```python
from build123d import *

# Parameters (mm, degrees)
SKETCH2_W           = 7.05
SKETCH2_H           = 26.75
BOSS_EXTRUDE1_DEPTH = 3.175
SKETCH3_W           = 7.05
SKETCH3_H           = 3.175
BOSS_EXTRUDE2_DEPTH = 20
SKETCH4_R           = 2.25
CUT_EXTRUDE1_DEPTH  = 3.175
SKETCH5_R           = 2.15
CUT_EXTRUDE2_DEPTH  = 34.585534461


with BuildPart() as part:
    # Sketch2 → Boss-Extrude1 (new body)
    with BuildSketch(Plane(origin=(0, 0, 0), x_dir=(1, 0, 0), z_dir=(0, 1, 0))):
        Rectangle(SKETCH2_W, SKETCH2_H)
    extrude(amount=BOSS_EXTRUDE1_DEPTH)

    # Sketch3 → Boss-Extrude2 (add)
    with BuildSketch(Plane.XZ):
        with Locations((0, 11.7875)):
            Rectangle(SKETCH3_W, SKETCH3_H)
        with Locations((0, -11.7875)):
            Rectangle(SKETCH3_W, SKETCH3_H)
    extrude(amount=BOSS_EXTRUDE2_DEPTH)

    # Sketch4 → Cut-Extrude1 (cut)
    with BuildSketch(Plane(origin=(0, 3.175, 0), x_dir=(1, 0, 0), z_dir=(0, 1, 0))):
        with Locations(Location((0, 5, 0), (0, 0, 270))):
            Circle(SKETCH4_R)
        with Locations(Location((0, -5, 0), (0, 0, 270))):
            Circle(SKETCH4_R)
    extrude(amount=-CUT_EXTRUDE1_DEPTH, mode=Mode.SUBTRACT)

    # Sketch5 → Cut-Extrude2 (cut, through all)
    with BuildSketch(Plane(origin=(0, 0, -13.375), x_dir=(-1, 0, 0), z_dir=(0, 0, -1))):
        with Locations((0, -7.825)):
            Circle(SKETCH5_R)
        with Locations((0, -15.825)):
            Circle(SKETCH5_R)
    extrude(amount=-CUT_EXTRUDE2_DEPTH, mode=Mode.SUBTRACT)


solid = part.part
```
Build history of the part. All positions in model axes, mm. A direction names the side the tool comes from. Give positions to 0.01 mm unless a question says otherwise; leave off trailing zeros. Loops run counter-clockwise (first coordinate to the right, second up) from the corner with the lowest first, then second, coordinate; pieces in that order, holes last. Notation, with made-up numbers: (42, 17) - (60, 17) arc R22 ccw to (60, 38) - close; hole circle Ø7 at (62, 80). An arc over 180 degrees is marked (long way). Use a Markdown table: item, result.
(1) Wall check: line 1 along Z through (x, y) = (-2.5, -0.75) (3 decimals); line 2 along Y through (x, z) = (1, 11.25) (3 decimals); line 3 along Y through (x, z) = (2.75, 2.25) (3 decimals). Give the ranges that are in metal, low to high.
Taken from the geometry:
| item | result |
|---|---|
| line 1 | -13.375 to -10.2, 10.2 to 13.375 |
| line 2 | -20 to -17.728, -13.922 to -9.728, -5.922 to 3.175 |
| line 3 | 0 to 3.175 |
(2) Band-saw the part on C-C (x = 0). Give the number of separate pieces and of enclosed holes in the cut face, and give its area (3 significant figures).
Taken from the geometry:
| item | result |
|---|---|
| separate pieces | 7 |
| enclosed holes | 0 |
| area | 129 mm2 |
(3) Band-saw the part on A-A (z = -5). Give the cut face in (x, y) (3 decimals), and give its area (3 significant figures).
Taken from the geometry:
| item | result |
|---|---|
| outline | (-3.525, 0) - (-2.25, 0) - (-2.25, 3.175) - (-3.525, 3.175) - close; (2.25, 0) - (3.525, 0) - (3.525, 3.175) - (2.25, 3.175) - close |
| area | 8.10 mm2 |
(4) Which spindle directions (+Z, -Z, +X, -X, +Y, -Y) get a long thin tool onto all of the face, cutting with end or side? Do faces 1 (the face through (-1, -10, -10.2)), 2 (the face through (-0.833, -5.675, 13.375)). Say none if no direction does.
Taken from the geometry:
| item | result |
|---|---|
| face 1 | +X, -X, -Y |
| face 2 | +Z, +X, -X, +Y, -Y |
(5) Pull direction X, two halves, no side cores. Call faces 3 (the face through (-1, -10, 10.2)), 4 (the face through (3.525, 0.2, -0.1)), 5 (the face through (-3.525, 0.2, -0.1)), 6 (the face through (1.585, -6.372, -11.81)): +X half, -X half, draft (parallel to the pull), parting line (faces both ways), or undercut.
Taken from the geometry:
| item | result |
|---|---|
| face 3 | draft |
| face 4 | +X half |
| face 5 | -X half |
| face 6 | undercut |
(6) Band-saw the part on B-B (y = -18.5). Give the cut face in (x, z) (3 decimals).
Taken from the geometry:
| item | result |
|---|---|
| outline | (-3.525, -13.375) - (3.525, -13.375) - (3.525, -10.2) - (-3.525, -10.2) - close; (-3.525, 10.2) - (3.525, 10.2) - (3.525, 13.375) - (-3.525, 13.375) - close |
(7) Band-saw the part on D-D (y = -6). Give the cut face in (x, z) (3 decimals).
Taken from the geometry:
| item | result |
|---|---|
| outline | (-3.525, -13.375) - (-1.137, -13.375) - (-1.137, -10.2) - (-3.525, -10.2) - close; (-3.525, 10.2) - (-1.137, 10.2) - (-1.137, 13.375) - (-3.525, 13.375) - close; (1.137, -13.375) - (3.525, -13.375) - (3.525, -10.2) - (1.137, -10.2) - close; (1.137, 10.2) - (3.525, 10.2) - (3.525, 13.375) - (1.137, 13.375) - close |
